```python
from build123d import *

# Parameters (mm, degrees)
SKETCH1_W                       = 46
SKETCH1_H                       = 40
BOSS_EXTRUDE1_DEPTH             = 21
CUT_EXTRUDE1_DEPTH              = 3
FILLET1_R                       = 8
SKETCH20_R                      = 40
BOSS_EXTRUDE3_DEPTH             = 4
M5_CLEARANCE_HOLE2_D            = 5.3
CIRPATTERN3_COUNT               = 4
SKETCH24_R                      = 14
CUT_EXTRUDE2_DEPTH              = 61.695963622
SKETCH25_R                      = 15
CUT_EXTRUDE3_DEPTH              = 12
M3X0_5_TAPPED_HOLE1_D           = 2.5
CIRPATTERN4_COUNT               = 4
CBORE_FOR_M4_SBHCS1_D           = 4.3
CBORE_FOR_M4_SBHCS1_CBORE_D     = 7.5
CBORE_FOR_M4_SBHCS1_CBORE_DEPTH = 5
FILLET2_R                       = 1
FILLET3_R                       = 0.5
FILLET4_R                       = 0.5


with BuildPart() as part:
    # Sketch1 → Boss-Extrude1 (new body)
    with BuildSketch(Plane.XY):
        Rectangle(SKETCH1_W, SKETCH1_H)
    extrude(amount=BOSS_EXTRUDE1_DEPTH)

    # Sketch2 → Cut-Extrude1 (cut)
    with BuildSketch(Plane(origin=(0, 0, 0), x_dir=(-1, 0, 0), z_dir=(0, 0, -1))):
        with BuildLine():
            Line((-23, -12), (-12.737739203, -12))
            ThreePointArc((-12.737739203, -12), (-9.62821501, -14.613263692), (-6, -16.439282223))
            Line((-6, -16.439282223), (-6, -20))
            Line((-6, -20), (6, -20))
            Line((6, -20), (6, -16.439282223))
            ThreePointArc((6, -16.439282223), (9.62821501, -14.613263692), (12.737739203, -12))
            Line((12.737739203, -12), (23, -12))
            Line((23, -12), (23, 12))
            Line((23, 12), (12.737739203, 12))
            ThreePointArc((12.737739203, 12), (9.62821501, 14.613263692), (6, 16.439282223))
            Line((6, 16.439282223), (6, 20))
            Line((6, 20), (-6, 20))
            Line((-6, 20), (-6, 16.439282223))
            ThreePointArc((-6, 16.439282223), (-9.62821501, 14.613263692), (-12.737739203, 12))
            Line((-12.737739203, 12), (-23, 12))
            Line((-23, 12), (-23, -12))
        make_face()
    extrude(amount=-CUT_EXTRUDE1_DEPTH, mode=Mode.SUBTRACT)

    # Fillet1
    fillet1_edges = [part.edges().sort_by_distance(p)[0] for p in [
        (-23, -20, 10.5),
        (23, -20, 10.5),
        (-23, 20, 10.5),
        (23, 20, 10.5),
    ]]
    fillet(fillet1_edges, radius=FILLET1_R)

    # Sketch20 → Boss-Extrude3 (add)
    with BuildSketch(Plane.XY.offset(21)):
        Circle(SKETCH20_R)
    extrude(amount=BOSS_EXTRUDE3_DEPTH)

    # M5 Clearance Hole2 (through all)
    with Locations(Plane.XY.offset(25)):
        with Locations((-36, 0)):
            m5_clearance_hole2 = Hole(M5_CLEARANCE_HOLE2_D / 2)

    # CirPattern3: M5 Clearance Hole2 ×4 about axis
    cirpattern3_axis = Axis((0, 0, 0), (0, 0, 1))
    for i in range(1, CIRPATTERN3_COUNT):
        add(m5_clearance_hole2.rotate(cirpattern3_axis, i * 360 / CIRPATTERN3_COUNT), mode=Mode.SUBTRACT)

    # Sketch24 → Cut-Extrude2 (cut, through all)
    with BuildSketch(Plane(origin=(0, 0, 3), x_dir=(-1, 0, 0), z_dir=(0, 0, -1))):
        Circle(SKETCH24_R)
    extrude(amount=-CUT_EXTRUDE2_DEPTH, mode=Mode.SUBTRACT)

    # Sketch25 → Cut-Extrude3 (cut)
    with BuildSketch(Plane.XY.offset(25)):
        Circle(SKETCH25_R)
    extrude(amount=-CUT_EXTRUDE3_DEPTH, mode=Mode.SUBTRACT)

    # M3x0.5 Tapped Hole1 (through all)
    with Locations(Plane(origin=(0, 0, 21), x_dir=(-1, 0, 0), z_dir=(0, 0, -1))):
        with Locations((23.140353949, 27.577599952), (27.577599952, 23.140353949)):
            m3x0_5_tapped_hole1 = Hole(M3X0_5_TAPPED_HOLE1_D / 2)

    # CirPattern4: M3x0.5 Tapped Hole1 ×4 about axis
    cirpattern4_axis = Axis((0, 0, 0), (0, 0, 1))
    for i in range(1, CIRPATTERN4_COUNT):
        add(m3x0_5_tapped_hole1.rotate(cirpattern4_axis, i * 360 / CIRPATTERN4_COUNT), mode=Mode.SUBTRACT)

    # CBORE for M4 SBHCS1 (through all)
    with Locations(Plane.XY.offset(25)):
        with Locations((-18, -8), (-18, 8), (18, -8), (18, 8)):
            CounterBoreHole(CBORE_FOR_M4_SBHCS1_D / 2, CBORE_FOR_M4_SBHCS1_CBORE_D / 2, CBORE_FOR_M4_SBHCS1_CBORE_DEPTH)

    # Fillet2
    fillet2_edges = [part.edges().sort_by_distance(p)[0] for p in [
        (0, -20, 21),
        (-23, 0, 21),
        (23, 0, 21),
        (0, 20, 21),
        (20.656854249, 17.656854249, 21),
        (-20.656854249, 17.656854249, 21),
        (20.656854249, -17.656854249, 21),
        (-20.656854249, -17.656854249, 21),
    ]]
    fillet(fillet2_edges, radius=FILLET2_R)

    # Fillet3
    fillet3_edges = [part.edges().sort_by_distance(p)[0] for p in [
        (6, 18.219641111, 3),
        (-9.62821501, 14.613263692, 3),
        (-17.868869601, 12, 3),
        (-9.62821501, -14.613263692, 3),
        (-6, -18.219641111, 3),
        (9.62821501, -14.613263692, 3),
        (17.868869601, -12, 3),
        (17.868869601, 12, 3),
        (9.62821501, 14.613263692, 3),
        (-6, 18.219641111, 3),
        (-17.868869601, -12, 3),
        (6, -18.219641111, 3),
    ]]
    fillet(fillet3_edges, radius=FILLET3_R)

    # Fillet4
    fillet4_edges = [part.edges().sort_by_distance(p)[0] for p in [
        (-15, 0, 13),
    ]]
    fillet(fillet4_edges, radius=FILLET4_R)


solid = part.part
```
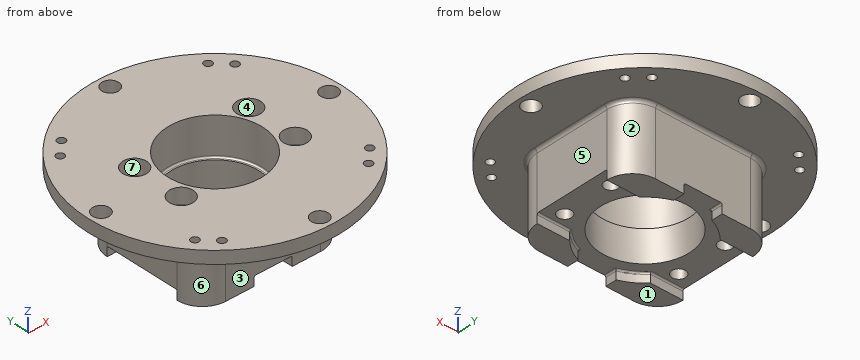
Work out the finished part from the listing and answer in its coordinate system (mm). Face numbers are marked on the shaded views. A direction names the side the tool comes from. Coordinates: 2 decimals unless noted, no trailing zeros. Loops run counter-clockwise (first coordinate to the right, second up) from the corner with the lowest first, then second, coordinate; pieces in that order, holes last. Notation, with made-up numbers: (20.25, 70.25) -> (40.25, 70.25) arc R11 ccw to (40.25, 88.25) -> close; hole circle Ø2 at (49, 14). An arc over 180 degrees is marked (long way). Answer as CSV lines item,"result".
Q1. The part is cut by section B-B on z = 15.75. Write down the section's boundary in (x, y).
Findings:
outline,"(-23, -12) arc R8 ccw to (-15, -20) -> (15, -20) arc R8 ccw to (23, -12) -> (23, 12) arc R8 ccw to (15, 20) -> (-15, 20) arc R8 ccw to (-23, 12) -> close; hole circle Ø4.3 at (-18, -8); hole circle Ø4.3 at (-18, 8); hole circle Ø30 at (0, 0); hole circle Ø4.3 at (18, -8); hole circle Ø4.3 at (18, 8)"
Q2. A tool of negligible diameter and unlimited length cuts with its end or side. For the marked faces 5, 6 and 7, from which of +Z, -Z, +X, -X, +Y, -Y can it reach the whole face along a straight path? Write none if from no direction.
Findings:
face 5,"-Z, +X, +Y, -Y"
face 6,"-Z, -X, -Y"
face 7,"+Z"
Q3. For a pull along Y with two mould halves and no side action, classify the marked faces 1, 2, 3 and 4 as +Y half, -Y half, draft (parallel to the pull), parting line (faces both ways), or undercut.
Findings:
face 1,"draft"
face 2,"+Y half"
face 3,"-Y half"
face 4,"undercut"
Q4. Each of these flat-tipped pins is pushed along its axis until it touches: pin 1 (4 mm diameter, centred on x = 23.14, y = -27.58, fed in from -Z); pin 2 (2 mm diameter, centred on x = -22, z = 14.5, fed in from +Y); pin 3 (5 mm diameter, centred on x = -18, y = 8, fed in from -Z). Where does it stop, or does it pass through?
Findings:
pin 1,"stops at z = 21"
pin 2,"stops at y = 17.29"
pin 3,"stops at z = 3"
Q5. Find the intervals of material crossed by probe 1 along Y at (x, z) = (-18, 8.75); probe 2 along Y at (x, z) = (0, 5.5); probe 3 along Z at (x, y) = (-13.5, 29), in increasing order.
Findings:
probe 1,"y = -19.42 to -10.15, -5.85 to 5.85, 10.15 to 19.42"
probe 2,"y = -20 to -14, 14 to 20"
probe 3,"z = 21 to 25"
Q6. The part is cut by section C-C on y = -36. Write down the section's boundary in (x, z), and give its area (3 significant figures).
Findings:
outline,"(-17.44, 21) -> (-2.65, 21) -> (-2.65, 25) -> (-17.44, 25) -> close; (2.65, 21) -> (17.44, 21) -> (17.44, 25) -> (2.65, 25) -> close"
area,"118 mm²"
Q7. The part is cut by section A-A on x = 0. Write down the section's boundary in (y, z).
Findings:
outline,"(-40, 21) -> (-38.65, 21) -> (-38.65, 25) -> (-40, 25) -> close; (-33.35, 21) -> (-21, 21) arc R1 cw to (-20, 20) -> (-20, 3) -> (-14, 3) -> (-14, 13) -> (-14.5, 13) arc R0.5 cw to (-15, 13.5) -> (-15, 25) -> (-33.35, 25) -> close; (14, 3) -> (20, 3) -> (20, 20) arc R1 cw to (21, 21) -> (33.35, 21) -> (33.35, 25) -> (15, 25) -> (15, 13.5) arc R0.5 cw to (14.5, 13) -> (14, 13) -> close; (38.65, 21) -> (40, 21) -> (40, 25) -> (38.65, 25) -> close"
